Source: three-view drawing plus pictorial views. Frame: mm from the lowest corner of the part. Round coordinates to 2 decimals unless told otherwise and drop trailing zeros. Loops run counter-clockwise (first coordinate to the right, second up) from the corner with the lowest first, then second, coordinate; pieces in that order, holes last. Notation, with made-up numbers: M 86,26.5 L 101,26.5 A15 cw 101,54.5 Z; hole C 1,11 d10. An arc over 180 degrees is marked long. Return JSON: item names as keys, results as strings. Group by question number.
1) Section A-A (x = 5.5). Output: boundary loops of the cut face in (y, z) (1 decimal).
2) Mould query, pull axis X, two halves, no side actions, for the marked faces 1, 2, 3 and 4. Classes: +X half, -X half, draft (parallel to the pull), parting line (faces both ways), or undercut.
3) Section D-D (y = 16.75). Output: boundary loops of the cut face in (x, z) (1 decimal).
4) Material intervals for line 1 (X direction, y = 8.75, z = 1.3) (1 decimal); line 2 (Y direction, x = 5.5, z = 1.6); line 3 (X direction, y = 9, z = 2.25) (1 decimal), sorted ascending. Write a range as from..to.
5) Section B-B (y = 9.5). Output: boundary loops of the cut face in (x, z) (1 decimal).
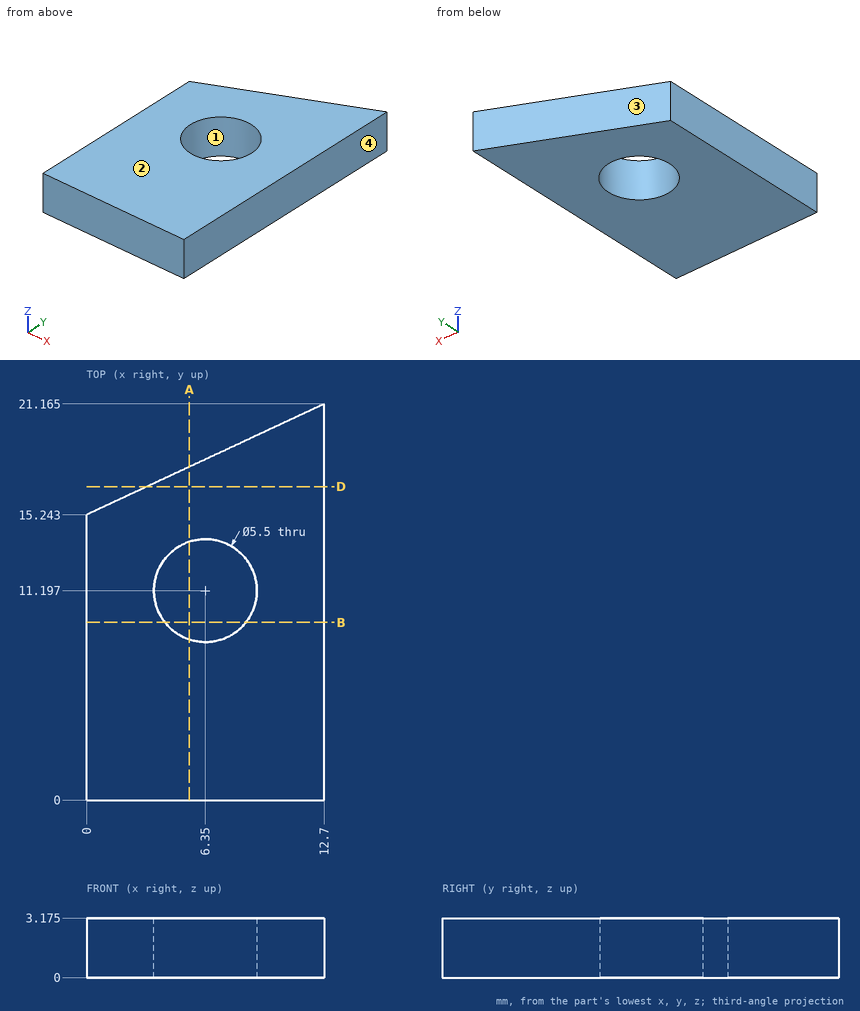
Returned:
{
 "1": {"outline": "M 0,0 L 8.6,0 L 8.6,3.2 L 0,3.2 Z; M 13.8,0 L 17.8,0 L 17.8,3.2 L 13.8,3.2 Z"},
 "2": {"face 1": "undercut", "face 2": "draft", "face 3": "-X half", "face 4": "+X half"},
 "3": {"outline": "M 3.2,0 L 12.7,0 L 12.7,3.2 L 3.2,3.2 Z"},
 "4": {"line 1": "x = 0..5.1, 7.6..12.7", "line 2": "y = 0..8.58, 13.81..17.81", "line 3": "x = 0..4.7, 8..12.7"},
 "5": {"outline": "M 0,0 L 4.2,0 L 4.2,3.2 L 0,3.2 Z; M 8.5,0 L 12.7,0 L 12.7,3.2 L 8.5,3.2 Z"}
}
